```python
from build123d import *

# Parameters (mm, degrees)
SKETCH_1_R               = 1.5
SKETCH_1_R_2             = 9
EXTRUDE_1_DEPTH          = 3
CHAMFER_1_SIZE           = 0.5
CUT_EXTRUDE_1_DEPTH      = 302.180394913
CUT_EXTRUDE_1_DEPTH_BACK = 302.180394913
SKETCH_3_R               = 1.5
CUT_EXTRUDE_2_DEPTH      = 302.180394913
CUT_EXTRUDE_2_DEPTH_BACK = 302.180394913
SKETCH_4_R               = 2
CHAMFER_2_SIZE           = 1
CUT_EXTRUDE_3_DEPTH      = 302.180394913
CUT_EXTRUDE_3_DEPTH_BACK = 302.180394913
SKETCH_5_R               = 1.5


with BuildPart() as part:
    # 草图1 → 凸台-拉伸1 (new body)
    with BuildSketch(Plane.XZ.offset(-78.025173071)):
        with BuildLine():
            Line((-212.541244563, -109.249486882), (-212.240178336, -124.096924988))
            ThreePointArc((-212.240178336, -124.096924988), (-212.661273384, -127.177841531), (-214.008389255, -129.980455778))
            ThreePointArc((-214.008389255, -129.980455778), (-174.628775953, -203.200190572), (-138.249712047, -128.44427297))
            ThreePointArc((-138.249712047, -128.44427297), (-139.709332875, -125.698571817), (-140.25497588, -122.637258129))
            Line((-140.25497588, -122.637258129), (-140.556042107, -107.789820023))
            ThreePointArc((-140.556042107, -107.789820023), (-141.477547023, -105.686749262), (-143.616244995, -104.85125604))
            Line((-143.616244995, -104.85125604), (-209.60268058, -106.189283994))
            ThreePointArc((-209.60268058, -106.189283994), (-211.705751342, -107.11078891), (-212.541244563, -109.249486882))
        make_face()
        with Locations((-136.648445194, -139.453062321)):
            Circle(SKETCH_1_R, mode=Mode.SUBTRACT)
        with Locations((-175.575532096, -156.509788424)):
            Circle(SKETCH_1_R_2, mode=Mode.SUBTRACT)
        with Locations((-135.988998284, -171.974468852)):
            Circle(SKETCH_1_R, mode=Mode.SUBTRACT)
        with Locations((-191.040212525, -196.096322235)):
            Circle(SKETCH_1_R, mode=Mode.SUBTRACT)
        with Locations((-215.162065908, -141.045107995)):
            Circle(SKETCH_1_R, mode=Mode.SUBTRACT)
        with Locations((-192.632258198, -117.582701522)):
            Circle(SKETCH_1_R, mode=Mode.SUBTRACT)
        with Locations((-160.110851668, -116.923254612)):
            Circle(SKETCH_1_R, mode=Mode.SUBTRACT)
        with Locations((-214.502618998, -173.566514526)):
            Circle(SKETCH_1_R, mode=Mode.SUBTRACT)
        with Locations((-158.518805994, -195.436875326)):
            Circle(SKETCH_1_R, mode=Mode.SUBTRACT)
    extrude(amount=EXTRUDE_1_DEPTH)

    # 倒角1
    chamfer_1_edges = [part.edges().sort_by_distance(p)[0] for p in [
        (-211.705751339, 75.025173077, -107.110788911),
        (-212.390711447, 75.025173077, -116.673205936),
        (-212.661273381, 75.025173077, -127.177841532),
        (-174.628775951, 75.025173075, -203.200190573),
        (-139.709332873, 75.025173075, -125.698571818),
        (-140.405508991, 75.025173075, -115.213539077),
        (-141.477547021, 75.025173075, -105.686749262),
        (-176.609462785, 75.025173076, -105.520270018),
    ]]
    chamfer(chamfer_1_edges, length=CHAMFER_1_SIZE)

    # 草图3 → 切除-拉伸1 (cut, two sides: drawn at the far end of the back side and taken through both)
    with BuildSketch(Plane.XZ.offset(-75.025173071).offset(-CUT_EXTRUDE_1_DEPTH_BACK)):
        with Locations((-200.041202679, -114.05266186)):
            Circle(SKETCH_3_R)
    extrude(amount=CUT_EXTRUDE_1_DEPTH + CUT_EXTRUDE_1_DEPTH_BACK, mode=Mode.SUBTRACT)

    # 草图4 → 切除-拉伸2 (cut, two sides: drawn at the far end of the back side and taken through both)
    with BuildSketch(Plane(origin=(2e-09, 78.025173071, -1e-09), x_dir=(1.0, -3.1446611841336594e-11, 0), z_dir=(3.1446611841336594e-11, 1.0, -6.574611909583631e-12)).offset(-CUT_EXTRUDE_2_DEPTH_BACK)):
        with Locations(Location((-192.064609975, 145.576946921, 0), (0, 0, 180))):
            Circle(SKETCH_4_R)
        with Locations(Location((-159.543203445, 144.917500011, 0), (0, 0, 180))):
            Circle(SKETCH_4_R)
        with Locations(Location((-187.634036488, 178.409388234, 0), (0, 0, 180))):
            Circle(SKETCH_4_R)
        with Locations(Location((-162.639174524, 177.902559463, 0), (0, 0, 180))):
            Circle(SKETCH_4_R)
    extrude(amount=CUT_EXTRUDE_2_DEPTH + CUT_EXTRUDE_2_DEPTH_BACK, mode=Mode.SUBTRACT)

    # 倒角2
    chamfer_2_edges = [part.edges().sort_by_distance(p)[0] for p in [
        (-212.390711447, 78.025173077, -116.673205936),
        (-211.705751339, 78.025173077, -107.110788911),
        (-176.609462785, 78.025173076, -105.520270018),
        (-141.477547021, 78.025173075, -105.686749262),
        (-184.575532094, 78.025173076, -156.509788424),
        (-140.405508991, 78.025173075, -115.213539077),
        (-139.709332873, 78.025173075, -125.698571818),
        (-174.62877595, 78.025173075, -203.200190573),
        (-212.661273381, 78.025173077, -127.177841532),
    ]]
    chamfer(chamfer_2_edges, length=CHAMFER_2_SIZE)

    # 草图5 → 切除-拉伸3 (cut, two sides: drawn at the far end of the back side and taken through both)
    with BuildSketch(Plane.XZ.offset(-75.025173071).offset(-CUT_EXTRUDE_3_DEPTH_BACK)):
        with Locations((-152.851097985, -113.09577309)):
            Circle(SKETCH_5_R)
    extrude(amount=CUT_EXTRUDE_3_DEPTH + CUT_EXTRUDE_3_DEPTH_BACK, mode=Mode.SUBTRACT)


solid = part.part
```
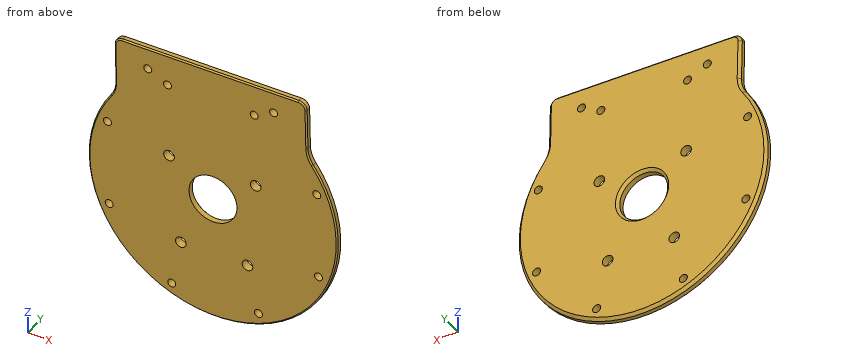
Model file for the job. Use its own axes, mm. Coordinates: 2 decimals unless noted, no trailing zeros. Use a Markdown table: item, result. Add a question column.
Item 1: Drill centre lines: line 1 along Z through (x, y) = (-137, 75.25); line 2 along X through (y, z) = (77.35, -188); line 3 along X through (y, z) = (75.6, -158.5). Where is each one in solid material? Low to high.
Item 2: Band-saw the part on A-A, the plane y = 76.25. Give the number of separate pieces and of enclosed holes in the cut face, and give its area (3 significant figures).
Item 3: Drop a flat-ended pin along its axis: pin 1 (1.5 mm diameter, centred on y = 75.5, z = -166.5, fed in from -X). Give the stop position or say it passes through.
A:
| question | item | result |
|---|---|---|
| 1 | line 1 | z = -182.34 to -173.08, -170.87 to -140.91, -137.99 to -130.68 |
| 1 | line 2 | x = -209.62 to -141.53 |
| 1 | line 3 | x = -222.23 to -184.35, -166.8 to -128.92 |
| 2 | separate pieces | 1 |
| 2 | enclosed holes | 15 |
| 2 | area | 7,160 mm² |
| 3 | pin 1 | stops at x = -221.35 |
